Check sheet for the modelled part. Datum: model origin and axes. Units: mm. A direction names the side the tool comes from. Round coordinates to 2 decimals unless told otherwise and drop trailing zeros. Write each loop counter-clockwise with the first axis right and the second up, starting at its lowest first coordinate (ties: lowest second). Pieces come first, ordered by that corner, then holes.
Item 1: Section check B-B, the plane z = 4. Record the cut outline in (x, y), plus the area to 3 significant figures.
Item 2: Material ranges on line 1 along Z through (x, y) = (-15.5, 3.5); line 2 along X through (y, z) = (-1.5, 6.75); line 3 along Y through (x, z) = (-17.5, 2.4), recorded low to high.
Item 3: Set-up check for faces 1 (the flat face through (-5.3, -3.2, 3.5)), 2 (the cylindrical face through (16.11, -1.06, 1.73)): record each of +Z, -Z, +X, -X, +Y, -Y from which the full face is reachable in a straight line by a thin tool's end or side.
Item 4: Release check for a two-part mould opening along Y. For faces 3 (the flat face through (-3, 1.8, 10)), 4 (the flat face through (3, -3, 13.5)), 5 (the cylindrical face through (-6, 0, 8)) record: pulls with the +Y half, pulls with the -Y half, needs draft (parallel to the pull), parting line crosses it, or undercut.
Item 5: Depth check by flat-ended pin: pin 1 (1 mm diameter, centred on x = -11, z = 2, fed in from -Y); pin 2 (4 mm diameter, centred on x = 3, z = 2, fed in from -Y); pin 3 (1 mm diameter, centred on x = -4, y = -5.5, fed in from +Z). Enter the tip coordinate at first touch or a pass-through.
Item 6: Section check A-A, the plane z = 9.25. Record the cut outline in (x, y).
from build123d import *

# Parameters (mm, degrees)
SKETCH1_RX          = 22.5
SKETCH1_RY          = 7.5
SKETCH1_R           = 1.75
BOSS_EXTRUDE2_DEPTH = 3.5
SKETCH3_R           = 6
BOSS_EXTRUDE3_DEPTH = 10
CUT_EXTRUDE5_DEPTH  = 7


with BuildPart() as part:
    # Sketch1 → Boss-Extrude2 (new body)
    with BuildSketch(Plane.XY):
        with Locations((0, 0)):
            Ellipse(SKETCH1_RX, SKETCH1_RY)
        with Locations((-17.5, 0)):
            Circle(SKETCH1_R, mode=Mode.SUBTRACT)
        with Locations((17.5, 0)):
            Circle(SKETCH1_R, mode=Mode.SUBTRACT)
    extrude(amount=BOSS_EXTRUDE2_DEPTH)

    # Sketch3 → Boss-Extrude3 (add)
    with BuildSketch(Plane.XY.offset(3.5)):
        Circle(SKETCH3_R)
    extrude(amount=BOSS_EXTRUDE3_DEPTH)

    # Sketch4 → Cut-Extrude5 (cut)
    with BuildSketch(Plane.XY.offset(13.5)):
        Polygon((4.041451884, 0), (2.020725942, 3.5), (-2.020725942, 3.5), (-4.041451884, 0), (-2.020725942, -3.5), (2.020725942, -3.5), align=None)
    extrude(amount=-CUT_EXTRUDE5_DEPTH, mode=Mode.SUBTRACT)


solid = part.part
Values found:
1. outline: circle Ø12 at (0, 0)
1. area: 113 mm2
2. line 1: z = 0 to 3.5
2. line 2: x = -5.81 to -3.18, 3.18 to 5.81
2. line 3: y = -4.71 to -1.75, 1.75 to 4.71
3. face 1: +Z
3. face 2: +Z, -Z
4. face 3: undercut
4. face 4: needs draft
4. face 5: parting line crosses it
5. pin 1: stops at y = -6.63
5. pin 2: stops at y = -7.49
5. pin 3: stops at z = 3.5
6. outline: circle Ø12 at (0, 0); hole (-4.04, 0) - (-2.02, -3.5) - (2.02, -3.5) - (4.04, 0) - (2.02, 3.5) - (-2.02, 3.5) - close
